Could you check a few things on this model? Use its own coordinates, in mm. A direction names the side the tool comes from. Give positions to 0.01 mm unless a question says otherwise; leave off trailing zeros. Order: outer loops, then holes, each group sorted by start corner. A loop starts at its lowest first (then second) coordinate and runs counter-clockwise, first axis right, second up. Notation, with made-up numbers: (-4, 84.25) -> (5, 84.25) arc R30 cw to (5, 106.25) -> close; hole circle Ø10 at (68.5, -25.75). An arc over 180 degrees is marked (long way). Write each question's results on one line, items separated by ' | '.
Autodesk Inventor part; units mm, degrees
ref_plane "YZ Plane" through (0, 0, 0) normal (1, 0, 0) x (0, 1, 0)
ref_plane "XZ Plane" through (0, 0, 0) normal (0, 1, 0) x (-1, 0, 0)
ref_plane "XY Plane" through (0, 0, 0) normal (0, 0, 1) x (1, 0, 0)
sketch "Sketch1" plane through (0, 0, 0) normal (0, 0, 1) x (1, 0, 0)
  circle A0 centre (0, -6) radius 1.1
  circle A1 centre (0, 6) radius 1.1
  circle A2 centre (-16, 13) radius 1.55
  circle A3 centre (16, 13) radius 1.55
  circle A4 centre (-16, -4.25) radius 1.55
  circle A5 centre (16, -4.25) radius 1.55
  arc A6 (17.7494, -6.7484) -> (16, -1.2) centre (16, -4.25) ccw
  arc A7 (12.9233, 1.4645) -> (16, -1.2) centre (16, 1.9085) ccw
  arc A8 (17.3284, 10.2545) -> (12.8667, 1.8571) centre (20.8351, 3.0073) ccw
  line L0 (12.9233, 1.4645) -> (12.8667, 1.8571)
  arc A9 (17.3284, 10.2545) -> (14.878, 15.8361) centre (16, 13) ccw
  arc A10 (-14.878, 15.8361) -> (14.878, 15.8361) centre (0, 53.4422) ccw
  arc A11 (-14.878, 15.8361) -> (-17.3284, 10.2545) centre (-16, 13) ccw
  arc A12 (-12.8667, 1.8571) -> (-17.3284, 10.2545) centre (-20.8351, 3.0073) ccw
  arc A13 (-16, -1.2) -> (-12.9233, 1.4645) centre (-16, 1.9085) ccw
  line L1 (-12.8667, 1.8571) -> (-12.9233, 1.4645)
  arc A14 (-16, -1.2) -> (-17.7494, -6.7484) centre (-16, -4.25) ccw
  line L2 (0, -6) -> (-7.5, -6) construction
  line L3 (-7.5, -6) -> (-7.5, 6) construction
  line L4 (-7.5, 6) -> (0, 6) construction
  line L5 (0, 6) -> (7.5, 6) construction
  line L6 (7.5, 6) -> (7.5, -6) construction
  line L7 (7.5, -6) -> (0, -6) construction
  arc A15 (-17.7494, -6.7484) -> (-16, -7.3) centre (-16, -4.25) ccw
  arc A16 (16, -1.2) -> (16, -7.3) centre (16, -4.25) ccw construction
  line L8 (-16, -7.3) -> (-7.5, -7.3)
  arc A17 (-0.875, -8.4483) -> (0.875, -8.4483) centre (0, -6) ccw
  arc A18 (7.5, -7.3) -> (0.875, -8.4483) centre (7.5, -26.9846) ccw
  arc A19 (-0.875, -8.4483) -> (-7.5, -7.3) centre (-7.5, -26.9846) ccw
  line L9 (-7.5, -7.3) -> (-2.2517, -7.3) construction
  line L10 (7.5, -7.3) -> (16, -7.3)
  arc A20 (-2.2517, -7.3) -> (-0.875, -8.4483) centre (0, -6) ccw construction
  arc A21 (0.875, -8.4483) -> (2.2517, -7.3) centre (0, -6) ccw construction
  arc A22 (2.2517, -7.3) -> (-2.2517, -7.3) centre (0, -6) ccw construction
  line L11 (-2.2517, -7.3) -> (2.2517, -7.3) construction
  line L12 (2.2517, -7.3) -> (7.5, -7.3) construction
  arc A23 (16, -7.3) -> (17.7494, -6.7484) centre (16, -4.25) ccw
  arc A24 (-16, -7.3) -> (-16, -1.2) centre (-16, -4.25) ccw construction
  point P0 (0, 0)
  dimension "d0" = 1.5
  dimension "d1" = 15
extrude "Extrusion1" add sketch "Sketch1" along normal blind 2.5
properties part number "AS5600_mount"
Q1. Suppose I cut it at A-A on x = 0. Please give me the cut outline in (y, z), and give its area (3 significant figures).
Here are the results:
outline: (-8.6, 0) -> (-7.1, 0) -> (-7.1, 2.5) -> (-8.6, 2.5) -> close; (-4.9, 0) -> (4.9, 0) -> (4.9, 2.5) -> (-4.9, 2.5) -> close; (7.1, 0) -> (13, 0) -> (13, 2.5) -> (7.1, 2.5) -> close | area: 43.0 mm²
Q2. For faces 4 (the cylindrical face through (-13.94, -0.42, 1.23)), 5 (the cylindrical face through (13.989, -0.462, 1.232)), 6 (the flat face through (-12, -7.3, 1)), which set-ups out of +Z, -Z, +X, -X, +Y, -Y let a thin tool reach every point of the face, with its end or its side?
Here are the results:
face 4: +Z, -Z, -X | face 5: +Z, -Z, +X | face 6: +Z, -Z, -X, -Y
Q3. Suppose I cut it at C-C on y = -4.25. Please give me the cut outline in (x, z).
Here are the results:
outline: (-19.05, 0) -> (-17.55, 0) -> (-17.55, 2.5) -> (-19.05, 2.5) -> close; (-14.45, 0) -> (14.45, 0) -> (14.45, 2.5) -> (-14.45, 2.5) -> close; (17.55, 0) -> (19.05, 0) -> (19.05, 2.5) -> (17.55, 2.5) -> close
Q4. Suppose I cut it at D-D on y = 6. Please give me the cut outline in (x, z).
Here are the results:
outline: (-13.36, 0) -> (-1.1, 0) -> (-1.1, 2.5) -> (-13.36, 2.5) -> close; (1.1, 0) -> (13.36, 0) -> (13.36, 2.5) -> (1.1, 2.5) -> close
Q5. Thinking about a two-plate mould opening in Y: for faces 1 (the flat face through (0, 4, 2.5)), 2 (the cylindrical face through (16.93, -7.155, 1.232)), 3 (the cylindrical face through (-18.925, -3.385, 1.232)), which applies, +Y half, -Y half, draft (parallel to the pull), parting line (faces both ways), or undercut?
Here are the results:
face 1: draft | face 2: -Y half | face 3: undercut
Q6. I'm going to push flat-ended pins straight in: pin 1 Ø1.5 at (x, z) = (3, 1) entering from +Y; pin 2 Ø1.5 at (x, z) = (-13, 0.5) entering from +Y. Where does each tip first touch, or does it pass through?
Here are the results:
pin 1: stops at y = 13.17 | pin 2: stops at y = 15.41
Q7. Suppose I cut it at B-B on z = 1.4. State how many separate pieces and enclosed holes the cut face has, and give its area (3 significant figures).
Here are the results:
separate pieces: 1 | enclosed holes: 6 | area: 661 mm²
Q8. I need wall thicknesses on line 1 along X through (y, z) = (-3, 0.6); line 2 along X through (y, z) = (-4, 1.9); line 3 along Y through (x, z) = (16, 1.4). Which ranges of each line are inside material? Lowest first, please.
Here are the results:
line 1: x = -18.78 to -16.92, -15.08 to 15.08, 16.92 to 18.78 | line 2: x = -19.04 to -17.53, -14.47 to 14.47, 17.53 to 19.04 | line 3: y = -7.3 to -5.8, -2.7 to -1.2, 9.44 to 11.45, 14.55 to 16.05
